```python
from build123d import *

# Parameters (mm, degrees)
SKETCH_4_W          = 0.8
SKETCH_4_H          = 5.94447729
CUT_EXTRUDE_1_DEPTH = 10


with BuildPart() as part:
    # 草图2 → 旋转1 (revolve)
    with BuildSketch(Plane.XY, mode=Mode.PRIVATE) as revolve_1_sk:
        Polygon((0, 0), (8, 0), (8, 0.299164486), (5.108022377, 4.7), (0, 4.7), align=None)
    revolve(revolve_1_sk.sketch.rotate(Axis((0, 6.286953345, 0), (0, -1, 0)), 90), axis=Axis((0, 6.286953345, 0), (0, -1, 0)))

    # 草图3 → 切除-旋转1 (revolve, cut)
    with BuildSketch(Plane.XY, mode=Mode.PRIVATE) as cut_revolve_1_sk:
        Polygon((1.2, 3.5), (1.2, 6.5), (0, 6.5), (0, 0), (7, 0), (4.7, 3.5), align=None)
    revolve(cut_revolve_1_sk.sketch.rotate(Axis((0, 5.949565502, 0), (0, -1, 0)), 90), axis=Axis((0, 5.949565502, 0), (0, -1, 0)), mode=Mode.SUBTRACT)

    # 草图4 → 切除-拉伸1 (cut)
    with BuildSketch(Plane.XY):
        with Locations((0, 2.524530629)):
            Rectangle(SKETCH_4_W, SKETCH_4_H)
    extrude(amount=-CUT_EXTRUDE_1_DEPTH, mode=Mode.SUBTRACT)


solid = part.part
```
Source: CAD feature listing. Evaluate the final solid. Frame: model axes, mm. A direction names the side the tool comes from. Give positions to 0.01 mm unless a question says otherwise; leave off trailing zeros. Loops run counter-clockwise (first coordinate to the right, second up) from the corner with the lowest first, then second, coordinate; pieces in that order, holes last. Notation, with made-up numbers: (32, -38.5) -> (61, -38.5) arc R24 ccw to (61, -16.5) -> close; hole circle Ø1 at (34, 14.5). An arc over 180 degrees is marked (long way). Use a Markdown table: item, result. Add a question column.
(1) Section query C-C (y = 2.45). Output: boundary loops of the cut face in (x, z), then the cut area to 3 significant figures.
(2) Ray query, line 1 (Z direction, x = 2.75, y = 1.15); line 2 (Y direction, x = 0.5, z = 1.25); line 3 (X direction, y = 3.95, z = 0). Return the intervals inside material, ascending.
(3) Pull-direction query (X, two-part tool) for faces 1 (the face through (0.4, 4, -5)), 2 (the face through (7.1, 0, -1.1)); classes: +X half, -X half, draft (parallel to the pull), parting line (faces both ways), or undercut.
(4) Access query for faces 3 (the face through (0, 4.1, 1.2)), 4 (the face through (-0.4, 4, -5)), 5 (the face through (1, 3.5, 1)). Directions: +Z, -Z, +X, -X, +Y, -Y. A direction counts if a zero-diameter tool reaches every point of the face in a straight line with its end or side. Return the directions, or none.
(5) First-contact query: pin 1 Ø3 at (x, z) = (-2, -2) entering from -Y; pin 2 Ø2.5 at (y, z) = (2, -5) entering from -X; pin 3 Ø2.5 at (y, z) = (3, -3.5) entering from +X; pin 4 Ø1.9 at (x, z) = (0, 0) entering from +Y. Flat tips, straight axial feed; report the tip coordinate or a pass-through.
(6) Section query B-B (y = 3.85). Output: boundary loops of the cut face in (x, z).
(7) Section query A-A (z = 0). Output: boundary loops of the cut face in (x, y), then the cut area to 3 significant figures.
Checked values:
| question | item | result |
|---|---|---|
| 1 | outline | (-0.4, -6.57) -> (-0.4, -5.38) arc R5.39 cw (long way) to (0.4, -5.38) -> (0.4, -6.57) arc R6.59 ccw (long way) to start |
| 1 | area | 44.1 mm^2 |
| 2 | line 1 | -6.91 to -5.61, 5.61 to 6.91 |
| 2 | line 2 | 3.5 to 4.7 |
| 2 | line 3 | -5.6 to -1.2, 1.2 to 5.6 |
| 3 | face 1 | undercut |
| 3 | face 2 | draft |
| 4 | face 3 | +Y, -Y |
| 4 | face 4 | -Z, +Y, -Y |
| 4 | face 5 | -Y |
| 5 | pin 1 | y = 3.5 |
| 5 | pin 2 | x = -6.23 |
| 5 | pin 3 | x = 6.31 |
| 5 | pin 4 | through |
| 6 | outline | (-0.4, -5.65) -> (-0.4, -1.13) arc R1.2 cw (long way) to (0.4, -1.13) -> (0.4, -5.65) arc R5.67 ccw (long way) to start |
| 7 | outline | (-8, 0) -> (-7, 0) -> (-4.7, 3.5) -> (-1.2, 3.5) -> (-1.2, 4.7) -> (-5.11, 4.7) -> (-8, 0.3) -> close; (1.2, 3.5) -> (4.7, 3.5) -> (7, 0) -> (8, 0) -> (8, 0.3) -> (5.11, 4.7) -> (1.2, 4.7) -> close |
| 7 | area | 18.6 mm^2 |
